CAD build for the part. Positions are in the model's coordinates, mm. A direction names the side the tool comes from. Coordinates: 2 decimals unless noted, no trailing zeros. Loops run counter-clockwise (first coordinate to the right, second up) from the corner with the lowest first, then second, coordinate; pieces in that order, holes last. Notation, with made-up numbers: M 88.25,-37 L 115.25,-37 A23 ccw 115.25,-13 Z; hole C 66,86.5 d3. An arc over 180 degrees is marked long. Answer as a JSON object with one key per item and string values. Group by question number.
```python
from build123d import *

# Parameters (mm, degrees)
F0_W     = 300
F0_H     = 50
F1_DEPTH = 12
F2_W     = 12
F2_H     = 15
F3_DEPTH = 12.5
F4_R     = 3
F5_DEPTH = 8
F6_R     = 3
F7_DEPTH = 12.001


with BuildPart() as f1:
    # F0 (on Top) → F1 (new body)
    with BuildSketch(Plane.XY):
        with Locations((-1.821462065, -2.0033000623)):
            Rectangle(F0_W, F0_H)
    extrude(amount=F1_DEPTH)

    # F2 (on face) → F3 (cut, symmetric)
    with BuildSketch(Plane.XY.offset(12)):
        with Locations((-145.821462065, 15.4966999377)):
            Rectangle(F2_W, F2_H)
        with Locations((-145.821462065, -19.5033000623)):
            Rectangle(F2_W, F2_H)
    extrude(amount=F3_DEPTH, both=True, mode=Mode.SUBTRACT)

    # F4 (on face) → F5 (cut)
    with BuildSketch(Plane.XY.offset(12)):
        with Locations((-33.821462065, -17.0033000623)):
            Circle(F4_R)
        with Locations((78.178537935, 12.9966999377)):
            Circle(F4_R)
        with Locations((78.178537935, -17.0033000623)):
            Circle(F4_R)
        with Locations((-33.821462065, 12.9966999377)):
            Circle(F4_R)
    extrude(amount=-F5_DEPTH, mode=Mode.SUBTRACT)

    # F6 (on face) → F7 (cut, through all)
    with BuildSketch(Plane.XY.offset(12)):
        with Locations((78.178537935, -2.0033000623)):
            Circle(F6_R)
    extrude(amount=-F7_DEPTH, mode=Mode.SUBTRACT)


solid = f1.part
```
Item 1: Tool access for faces 5 (the flat face through (2, -27.003, 6)), 6 (the flat face through (-139.821, -20, 6)), 7 (the flat face through (-139.821, 15, 6)), 8 (the flat face through (-34, 13, 4)): list every direction of +Z, -Z, +X, -X, +Y, -Y with a clear straight run to the whole face (end or side of a thin tool).
Item 2: Pull direction X, two halves, no side cores. Call faces 1 (the flat face through (-151.821, -2, 6)), 2 (the flat face through (-4, -2, 12)), 3 (the flat face through (78, -17, 4)), 4 (the flat face through (148.179, -2, 6)): released by +X, released by -X, zero draft, split by the parting line, or undercut.
Item 3: Slice it at A-A, the plane z = 2. Write the cut outline in (x, y).
Item 4: Drill centre lines: L1, parallel to X at y = -15, z = 6.75; L2, parallel to X at y = -12.5, z = 1.5; L3, parallel to X at y = 0.5, z = 10.25. Where is each one in solid material? Low to high. Write a range as from..to.
Item 5: Pin check, flat tips, straight feed: pin 1 (6.5 mm diameter, centred on x = 79.5, y = -16.5, fed in from +Z); pin 2 (5.5 mm diameter, centred on x = 78.18, y = -17, fed in from +Z); pin 3 (3.5 mm diameter, centred on x = -146, z = 5, fed in from +Y); pin 4 (6 mm diameter, centred on y = -16.5, z = 9, fed in from -X). Stop position of each tip, or through.
Computed:
{
 "1": {"face 5": "+Z, -Z, +X, -X, -Y", "face 6": "+Z, -Z, -X, -Y", "face 7": "+Z, -Z, -X, +Y", "face 8": "+Z"},
 "2": {"face 1": "released by -X", "face 2": "zero draft", "face 3": "undercut", "face 4": "released by +X"},
 "3": {"outline": "M -151.82,-12 L -139.82,-12 L -139.82,-27 L 148.18,-27 L 148.18,23 L -139.82,23 L -139.82,8 L -151.82,8 Z; hole C 78.18,-2 d6"},
 "4": {"L1": "-139.82..-36.05, -31.59..75.95, 80.41..148.18", "L2": "-139.82..148.18", "L3": "-151.82..76.53, 79.83..148.18"},
 "5": {"pin 1": "z = 12", "pin 2": "z = 4", "pin 3": "y = 8", "pin 4": "x = -139.82"}
}
